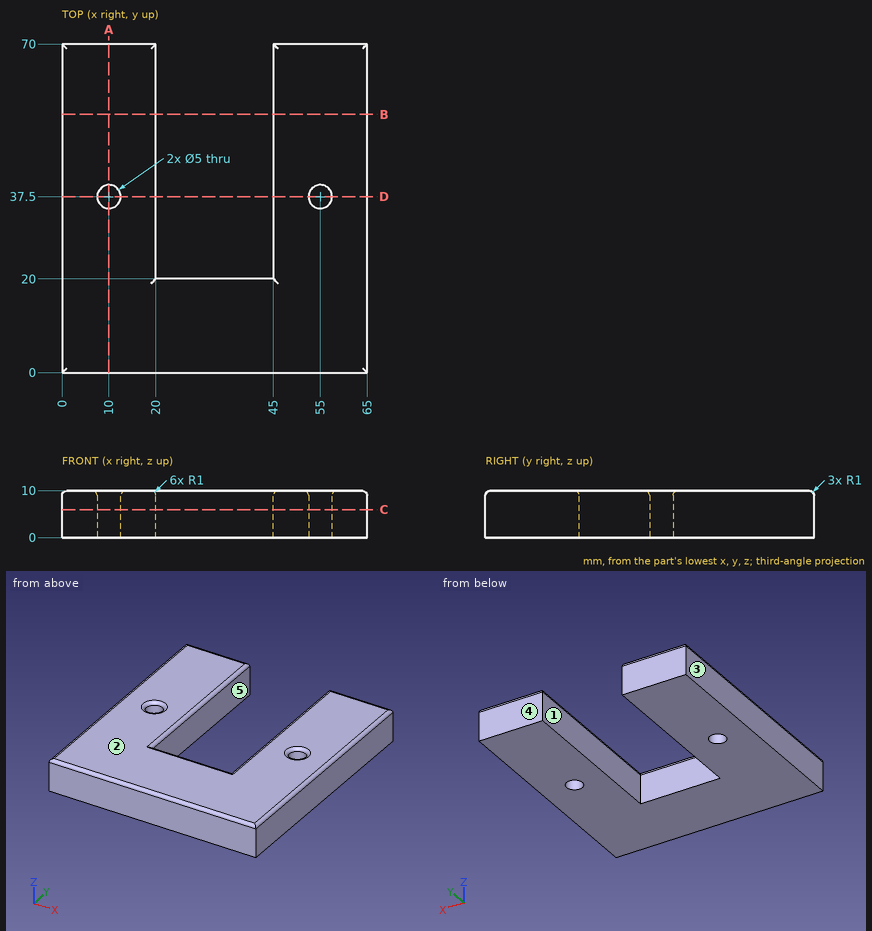
Verification items for this drawing (mm, ordinates from the low corner). A direction names the side the tool comes from. Give positions to 0.01 mm unless a question says otherwise; leave off trailing zeros. Loops run counter-clockwise (first coordinate to the right, second up) from the corner with the lowest first, then second, coordinate; pieces in that order, holes last. Notation, with made-up numbers: M 69.25,6 L 120.25,6 A18 cw 120.25,34 Z; hole C 64,56 d5. An arc over 180 degrees is marked long. Answer as CSV lines item,"result".
Item 1: Material ranges on line 1 (X direction, y = 38.5, z = 6); line 2 (X direction, y = 41, z = 4.5); line 3 (Y direction, x = 55, z = 6), recorded low to high.
Values:
line 1,"x = 0 to 7.71, 12.29 to 20, 45 to 52.71, 57.29 to 65"
line 2,"x = 0 to 20, 45 to 65"
line 3,"y = 0 to 35, 40 to 70"
Item 2: Cross-section at B-B on y = 55. Record the cut outline in (x, z).
Values:
outline,"M 0,0 L 20,0 L 20,9 A1 ccw 19,10 L 1,10 A1 ccw 0,9 Z; M 45,0 L 65,0 L 65,9 A1 ccw 64,10 L 46,10 A1 ccw 45,9 Z"
Item 3: Cross-section at C-C on z = 6. Record the cut outline in (x, y).
Values:
outline,"M 0,0 L 65,0 L 65,70 L 45,70 L 45,20 L 20,20 L 20,70 L 0,70 Z; hole C 10,37.5 d5; hole C 55,37.5 d5"
Item 4: Release check for a two-part mould opening along X. For the marked faces 1, 2 and 3 record: pulls with the +X half, pulls with the -X half, needs draft (parallel to the pull), parting line crosses it, or undercut.
Values:
face 1,"undercut"
face 2,"needs draft"
face 3,"pulls with the -X half"
Item 5: Cross-section at A-A on x = 10. Record the cut outline in (y, z), and give its area (3 significant figures).
Values:
outline,"M 0,0 L 35,0 L 35,9 A1 ccw 34,10 L 1,10 A1 ccw 0,9 Z; M 40,0 L 70,0 L 70,9 A1 ccw 69,10 L 41,10 A1 ccw 40,9 Z"
area,"649 mm²"
Item 6: Cross-section at D-D on y = 37.5. Record the cut outline in (x, z), and give its area (3 significant figures).
Values:
outline,"M 0,0 L 7.5,0 L 7.5,9 A1 ccw 6.5,10 L 1,10 A1 ccw 0,9 Z; M 12.5,0 L 20,0 L 20,9 A1 ccw 19,10 L 13.5,10 A1 ccw 12.5,9 Z; M 45,0 L 52.5,0 L 52.5,9 A1 ccw 51.5,10 L 46,10 A1 ccw 45,9 Z; M 57.5,0 L 65,0 L 65,9 A1 ccw 64,10 L 58.5,10 A1 ccw 57.5,9 Z"
area,"298 mm²"
Item 7: Depth check by flat-ended pin: P1, Ø4, axis at x = 55, y = 37.5, coming from the -Z side; P2, Ø2.5, axis at x = 35, z = 3, coming from the +Y side; P3, Ø1, axis at x = 56, y = 45.5, coming from the -Z side. Enter the tip coordinate at first touch or a pass-through.
Values:
P1,"passes through"
P2,"stops at y = 20"
P3,"stops at z = 0"
Item 8: Access from +Z, -Z, +X, -X, +Y, -Y to the whole of each face (thin tool, end or side, straight path). Record for the marked faces 4 and 5.
Values:
face 4,"+Z, -Z, +X, -X, +Y"
face 5,"+Z, -Z, +Y"
